Design review of the part built by this model. Coordinates are the model's own, in mm. A direction names the side the tool comes from. Give positions to 0.01 mm unless a question says otherwise; leave off trailing zeros. Loops run counter-clockwise (first coordinate to the right, second up) from the corner with the lowest first, then second, coordinate; pieces in that order, holes last. Notation, with made-up numbers: (72, 71.25) -> (114, 71.25) arc R31 ccw to (114, 109.25) -> close; hole circle Ø2 at (-26, 79.25). An arc over 180 degrees is marked (long way). Use CSV: the item, a comma, the result in double quotes. Start each with the question number.
Item 1: The part is to be moulded in two halves that separate along Z. For faces 1 (the face through (6.466, 15.196, 2.681)), 2 (the face through (6.8, 10, -10.7)), 3 (the face through (14.985, 4.549, -0.66)), say which applies: +Z half, -Z half, draft (parallel to the pull), parting line (faces both ways), or undercut.
Item 2: We need section A-A (x = 0). State the section outline as (y, z) points, plus the area to 3 significant figures.
Item 3: We need section B-B (y = 7.5). State the section outline as (x, z) points, plus the area to 3 significant figures.
Item 4: We need section C-C (y = 15.25). State the section outline as (x, z) points, plus the area to 3 significant figures.
Item 5: Clearance check with flat-ended pins moving along their axes: pin 1 (8.5 mm diameter, centred on x = 0, z = 0, fed in from -Y); pin 2 (10 mm diameter, centred on x = 10.5, y = 7, fed in from +Z); pin 3 (6 mm diameter, centred on x = -9, y = 11, fed in from +Z); pin 4 (4 mm diameter, centred on y = 14, z = -3, fed in from +X). State where each tip first meets the part, or that it passes through.
Item 6: For faces 4 (the face through (-11.923, 19.633, -3.755)), 5 (the face through (6, 0, 6)), list the 3-axis set-ups (+Z, -Z, +X, -X, +Y, -Y) from which the entire face can be reached by the end or side of a thin tool; tool diameter is ignored.
Item 7: Wall thickness on line 1 along Z through (x, y) = (0, 13.75); line 2 along Z through (x, y) = (0, 7.5): over which ranges is each line inside the solid? List them lowest first. Write a range as from..to.
from build123d import *

# Parameters (mm, degrees)
CHAMFER_1_SIZE         = 1
CHAMFER_2_SIZE         = 2
HOLE_WIZARD_M161_D     = 14
HOLE_WIZARD_M161_DEPTH = 50
HOLE_WIZARD_M161_TIP   = 4.041451884
CHAMFER_3_SIZE         = 1


with BuildPart() as part:
    # Эскиз1 → Повернуть1 (revolve)
    with BuildSketch(Plane.XY):
        Polygon((0, 0), (-15, 0), (-15, 10), (-12.5, 10), (-12.5, 30), (0, 30), align=None)
    revolve(axis=Axis((0, 30, 0), (0, -1, 0)))

    # Фаска1
    chamfer_1_edges = [part.edges().sort_by_distance(p)[0] for p in [
        (12.5, 30, 0),
        (15, 0, 0),
    ]]
    chamfer(chamfer_1_edges, length=CHAMFER_1_SIZE)

    # Фаска2
    chamfer_2_edges = [part.edges().sort_by_distance(p)[0] for p in [
        (15, 10, 0),
    ]]
    chamfer(chamfer_2_edges, length=CHAMFER_2_SIZE)

    # Отверстие обработанное метчиком M161
    with Locations(Plane(origin=(0, 0, 0), x_dir=(-1, 0, 0), z_dir=(0, -1, 0))):
        with Locations((0, 0)):
            Hole(HOLE_WIZARD_M161_D / 2, depth=HOLE_WIZARD_M161_DEPTH)
            with Locations((0, 0, -(HOLE_WIZARD_M161_DEPTH + HOLE_WIZARD_M161_TIP / 2))):  # 120° drill point
                Cone(0, HOLE_WIZARD_M161_D / 2, HOLE_WIZARD_M161_TIP, mode=Mode.SUBTRACT)

    # Фаска3
    chamfer_3_edges = [part.edges().sort_by_distance(p)[0] for p in [
        (-7, 30, 0),
        (-7, 0, 0),
    ]]
    chamfer(chamfer_3_edges, length=CHAMFER_3_SIZE)


solid = part.part
Results found:
1,face 1,"undercut"
1,face 2,"draft"
1,face 3,"parting line"
2,outline,"(0, -14) -> (1, -15) -> (8, -15) -> (10, -13) -> (10, -12.5) -> (29, -12.5) -> (30, -11.5) -> (30, -8) -> (29, -7) -> (1, -7) -> (0, -8) -> close; (0, 8) -> (1, 7) -> (29, 7) -> (30, 8) -> (30, 11.5) -> (29, 12.5) -> (10, 12.5) -> (10, 13) -> (8, 15) -> (1, 15) -> (0, 14) -> close"
2,area,"372 mm²"
3,outline,"circle Ø30 at (0, 0); hole circle Ø14 at (0, 0)"
3,area,"553 mm²"
4,outline,"circle Ø25 at (0, 0); hole circle Ø14 at (0, 0)"
4,area,"337 mm²"
5,pin 1,"through"
5,pin 2,"z = 13.96"
5,pin 3,"z = 12.53"
5,pin 4,"x = 12.46"
6,face 4,"+Y"
6,face 5,"+Z, -Z, +X, -X, -Y"
7,line 1,"-12.5..-7, 7..12.5"
7,line 2,"-15..-7, 7..15"
